CAD build for the part. Positions are in the model's coordinates, mm. A direction names the side the tool comes from. Give positions to 0.01 mm unless a question says otherwise; leave off trailing zeros. Write each loop counter-clockwise with the first axis right and the second up, starting at its lowest first coordinate (ties: lowest second). Pieces come first, ordered by that corner, then holes. Notation, with made-up numbers: (72, 15) - (81, 15) arc R10 ccw to (81, 25) - close; hole circle Ø7 at (-2.5, 11). An arc over 180 degrees is marked (long way). Answer as a JSON object with one key per item and string values.
from build123d import *

# Parameters (mm, degrees)
F1_DEPTH = 24
F2_R     = 2
F3_R     = 1.8
F4_DEPTH = 30.001
F5_R     = 5
F7_DEPTH = 23.001


with BuildPart() as f1:
    # F0 (on Front) → F1 (new body)
    with BuildSketch(Plane.XZ):
        Polygon((-30, 0), (0, 0), (0, 23), (-3, 23), (-3, 3), (-30, 3), align=None)
    extrude(amount=F1_DEPTH)

    # F2
    f2_edges = [f1.edges().sort_by_distance(p)[0] for p in [
        (-3, -12, 3),
    ]]
    fillet(f2_edges, radius=F2_R)

    # F3 (on face) → F4 (cut, through all)
    with BuildSketch(Plane.YZ):
        with Locations((-12, 15)):
            Circle(F3_R)
    extrude(amount=-F4_DEPTH, mode=Mode.SUBTRACT)

    # F5
    f5_edges = [f1.edges().sort_by_distance(p)[0] for p in [
        (-1.5, -24, 23),
        (-1.5, 0, 23),
        (-30, -24, 1.5),
        (-30, 0, 1.5),
    ]]
    fillet(f5_edges, radius=F5_R)

    # F6 (on face) → F7 (cut, through all)
    with BuildSketch(Plane(origin=(0, 0, 0), x_dir=(1, 0, 0), z_dir=(0, 0, -1))):
        with BuildLine():
            ThreePointArc((-8, 18.25), (-6.25, 20), (-8, 21.75))
            Line((-8, 21.75), (-22, 21.75))
            ThreePointArc((-22, 21.75), (-23.75, 20), (-22, 18.25))
            Line((-22, 18.25), (-8, 18.25))
        make_face()
        with BuildLine():
            Line((-22, 2.25), (-8, 2.25))
            ThreePointArc((-8, 2.25), (-6.25, 4), (-8, 5.75))
            Line((-8, 5.75), (-22, 5.75))
            ThreePointArc((-22, 5.75), (-23.75, 4), (-22, 2.25))
        make_face()
    extrude(amount=-F7_DEPTH, mode=Mode.SUBTRACT)


solid = f1.part
Item 1: Mould opens along Y. For faces 1 (the cylindrical face through (-28, -23, 1)), 2 (the flat face through (-15, -2.25, 1)), 3 (the flat face through (-17, -12, 3)) say: +Y half, -Y half, draft (parallel to the pull), parting line (faces both ways), or undercut.
Entries:
{"face 1": "-Y half", "face 2": "undercut", "face 3": "draft"}
Item 2: Flat gauge pins, fed straight in: P1, Ø9, axis at y = -16, z = 11.5, coming from the -X side; P2, Ø1.5, axis at y = -5.5, z = 19.5, coming from the +X side; P3, Ø8, axis at x = -25, y = -18.5, coming from the +Z side. Where does each tip first touch, or does it go through?
Entries:
{"P1": "x = -3", "P2": "x = 0", "P3": "z = 3"}
Item 3: Cut at A-A (z = 15). Give the cut face in (x, y).
Entries:
{"outline": "(-3, -24) - (0, -24) - (0, -13.8) - (-3, -13.8) - close; (-3, -10.2) - (0, -10.2) - (0, 0) - (-3, 0) - close"}
Item 4: Cut at C-C (x = -10.75). Give the cut face in (y, z).
Entries:
{"outline": "(-24, 0) - (-21.75, 0) - (-21.75, 3) - (-24, 3) - close; (-18.25, 0) - (-5.75, 0) - (-5.75, 3) - (-18.25, 3) - close; (-2.25, 0) - (0, 0) - (0, 3) - (-2.25, 3) - close"}
Item 5: Probe line 1 (Z direction, x = -2.25, y = -12); line 2 (X direction, y = -4, z = 13.25); line 3 (Z direction, x = -16.25, y = -15). List the from-to ranges inside material, lowest first. Write a range as from..to.
Entries:
{"line 1": "0..13.2, 16.8..23", "line 2": "-3..0", "line 3": "0..3"}
Item 6: Cut at B-B (y = -12). Give the cut face in (x, z).
Entries:
{"outline": "(-30, 0) - (0, 0) - (0, 13.2) - (-3, 13.2) - (-3, 5) arc R2 cw to (-5, 3) - (-30, 3) - close; (-3, 16.8) - (0, 16.8) - (0, 23) - (-3, 23) - close"}
Item 7: Cut at D-D (y = -14.5). Give the cut face in (x, z), and give its area (3 significant figures).
Entries:
{"outline": "(-30, 0) - (0, 0) - (0, 23) - (-3, 23) - (-3, 5) arc R2 cw to (-5, 3) - (-30, 3) - close", "area": "151 mm2"}
Item 8: Which spindle directions (+Z, -Z, +X, -X, +Y, -Y) get a long thin tool onto all of the face, cutting with end or side? Do faces 4 (the cylindrical face through (-28, -1, 1)), 5 (the cylindrical face through (-6.25, -3.96, 1.48)). Say none if no direction does.
Entries:
{"face 4": "+Z, -Z, -X, +Y", "face 5": "+Z, -Z"}
